```python
from build123d import *

# Parameters (mm, degrees)
CYLINDER002_R          = 2
CYLINDER002_DEPTH      = 10
CYLINDER002_ROLL_ANGLE = -90
CYLINDER001_R          = 18.5
CYLINDER001_DEPTH      = 10
CYLINDER003_R          = 2
CYLINDER003_DEPTH      = 10
CYLINDER003_ROLL_ANGLE = -90
BOX_W                  = 40
BOX_H                  = 5
BOX_DEPTH              = 10
CYLINDER_R             = 22
CYLINDER_DEPTH         = 10


with BuildPart() as cylinder002:
    # Cylinder002 → Cylinder002 (new body)
    with BuildSketch(Plane.XY):
        Circle(CYLINDER002_R)
    extrude(amount=CYLINDER002_DEPTH)


with BuildPart() as cylinder002_1:
    # Cylinder002 roll: moved
    add(cylinder002.part.rotate(Axis((0, 0, 0), (1, 0, 0)), CYLINDER002_ROLL_ANGLE))


with BuildPart() as cylinder002_2:
    # Cylinder002 placement: moved
    add(cylinder002_1.part.moved(Location((15, 20, 0))))


with BuildPart() as cylinder001:
    # Cylinder001 → Cylinder001 (new body)
    with BuildSketch(Plane.XY.offset(-5)):
        Circle(CYLINDER001_R)
    extrude(amount=CYLINDER001_DEPTH)


with BuildPart() as negative_fusion:
    # Cylinder003 → Cylinder003 (new body)
    with BuildSketch(Plane.XY):
        Circle(CYLINDER003_R)
    extrude(amount=CYLINDER003_DEPTH)


with BuildPart() as negative_fusion_1:
    # Cylinder003 roll: moved
    add(negative_fusion.part.rotate(Axis((0, 0, 0), (1, 0, 0)), CYLINDER003_ROLL_ANGLE))


with BuildPart() as negative_fusion_2:
    # Cylinder003 placement: moved
    add(negative_fusion_1.part.moved(Location((-15, 20, 0))))

    # Fusion001: union Cylinder002, Cylinder001
    add(cylinder002_2.part)
    add(cylinder001.part)


with BuildPart() as cube:
    # Box → Box (new body)
    with BuildSketch(Plane(origin=(-20, 20, -5), x_dir=(1, 0, 0), z_dir=(0, 0, 1))):
        with Locations((20, 2.5)):
            Rectangle(BOX_W, BOX_H)
    extrude(amount=BOX_DEPTH)


with BuildPart() as cut:
    # Cylinder → Cylinder (new body)
    with BuildSketch(Plane.XY.offset(-5)):
        Circle(CYLINDER_R)
    extrude(amount=CYLINDER_DEPTH)

    # Fusion: union Cube
    add(cube.part)

    # Cut: cut Negative Fusion
    add(negative_fusion_2.part, mode=Mode.SUBTRACT)


solid = cut.part
```
Input: part model. Units: mm. Frame: model coordinates. A direction names the side the tool comes from. Coordinates: 2 decimals unless noted, no trailing zeros. Order: outer loops, then holes, each group sorted by start corner. A loop starts at its lowest first (then second) coordinate and runs counter-clockwise, first axis right, second up. Notation, with made-up numbers: (-31, 5.5) - (-17, 5.5) arc R16 ccw to (-17, 30.5) - close; hole circle Ø3 at (-8, 55). An arc over 180 degrees is marked (long way). Return JSON: item names as keys, results as strings.
Q1. Cut plane D-D (z = -3.75). Return loops of the section in (x, y), then the cut area to 3 significant figures.
The answers:
{"outline": "(-20, 20) - (-9.17, 20) arc R22 ccw (long way) to (9.17, 20) - (20, 20) - (20, 25) - (-20, 25) - close; hole circle Ø37 at (0, 0)", "area": "621 mm2"}
Q2. Cut plane A-A (y = 0). Return loops of the section in (x, z), then the cut area to 3 significant figures.
The answers:
{"outline": "(-22, -5) - (-18.5, -5) - (-18.5, 5) - (-22, 5) - close; (18.5, -5) - (22, -5) - (22, 5) - (18.5, 5) - close", "area": "70.0 mm2"}
Q3. Draft query along X for faces 1 (the flat face through (-20, 22, 0)), 2 (the flat face through (0, 19, -5)), 3 (the cylindrical face through (-16.6, 22.5, 1.2)). Return one class per face: +X half, -X half, draft (parallel to the pull), parting line (faces both ways), or undercut.
The answers:
{"face 1": "-X half", "face 2": "draft", "face 3": "undercut"}
Q4. Ray query, probe 1 along X at (y, z) = (21, 0); probe 2 along Y at (x, z) = (0, 1.5); probe 3 along Y at (x, z) = (15, 3.75). Return the intervals inside material, ascending.
The answers:
{"probe 1": "x = -20 to -17, -13 to 13, 17 to 20", "probe 2": "y = -22 to -18.5, 18.5 to 25", "probe 3": "y = -16.09 to -10.83, 10.83 to 16.09, 20 to 25"}
Q5. Access query for faces 4 (the flat face through (20, 22, 0)), 5 (the cylindrical face through (13.4, 22.5, 1.2)), 6 (the cylindrical face through (-4.01, -18.06, -0.07)). Directions: +Z, -Z, +X, -X, +Y, -Y. A direction counts if a zero-diameter tool reaches every point of the face in a straight line with its end or side. Return the directions, or none.
The answers:
{"face 4": "+Z, -Z, +X, +Y", "face 5": "+Y", "face 6": "+Z, -Z"}
Q6. First-contact query: pin 1 (3 mm diameter, centred on x = -14.5, z = 2, fed in from -Y); pin 2 (1.5 mm diameter, centred on y = 21.5, z = 1, fed in from -X); pin 3 (4 mm diameter, centred on y = 23.5, z = -1.5, fed in from +X); pin 4 (10 mm diameter, centred on x = 8.5, y = 13.5, fed in from -Z). Flat tips, straight axial feed; report the tip coordinate or a pass-through.
The answers:
{"pin 1": "stops at y = -17.75", "pin 2": "stops at x = -20", "pin 3": "stops at x = 20", "pin 4": "stops at z = -5"}
Q7. Cut plane B-B (z = 0). Return loops of the section in (x, y), then the cut area to 3 significant figures.
The answers:
{"outline": "(-20, 20) - (-17, 20) - (-17, 25) - (-20, 25) - close; (-13, 20) - (-9.17, 20) arc R22 ccw (long way) to (9.17, 20) - (13, 20) - (13, 25) - (-13, 25) - close; (17, 20) - (20, 20) - (20, 25) - (17, 25) - close; hole circle Ø37 at (0, 0)", "area": "581 mm2"}
Q8. Cut plane C-C (x = 0). Return loops of the section in (y, z).
The answers:
{"outline": "(-22, -5) - (-18.5, -5) - (-18.5, 5) - (-22, 5) - close; (18.5, -5) - (25, -5) - (25, 5) - (18.5, 5) - close"}
